from build123d import *

# Parameters (mm, degrees)
SKETCH1_R           = 0.5
SKETCH1_R_2         = 1.695720035
SKETCH1_W           = 3.739481929
SKETCH1_H           = 1.068423409
SKETCH1_W_2         = 3.73948193
BOSS_EXTRUDE1_DEPTH = 4


with BuildPart() as part:
    # Sketch1 → Boss-Extrude1 (new body)
    with BuildSketch(Plane(origin=(0, 0, 0), x_dir=(1, 0, 0), z_dir=(0, 1, 0))):
        with BuildLine():
            Line((43.455785529, -19.365174275), (43.455785529, 24.440185465))
            Line((43.455785529, 24.440185465), (39.576612996, 24.440185465))
            Line((39.576612996, 24.440185465), (39.576612996, 12.960768953))
            Line((39.576612996, 12.960768953), (19.950470546, 12.960768953))
            Line((19.950470546, 12.960768953), (19.950470546, 24.039526687))
            Line((19.950470546, 24.039526687), (-11.673190701, 24.438144265))
            ThreePointArc((-11.673190701, 24.438144265), (-5.411187986, 17.934763274), (-11.83512585, 11.591289096))
            Line((-11.83512585, 11.591289096), (-30.532535496, 11.591289096))
            ThreePointArc((-30.532535496, 11.591289096), (-36.95698368, 18.01573728), (-30.532535496, 24.440185465))
            Line((-30.532535496, 24.440185465), (-37.72291673, 24.440185465))
            Line((-37.72291673, 24.440185465), (-37.72291673, -19.365174275))
            Line((-37.72291673, -19.365174275), (-30.532535496, -19.365174275))
            ThreePointArc((-30.532535496, -19.365174275), (-37.109148108, -12.788561662), (-30.532535496, -6.21194905))
            Line((-30.532535496, -6.21194905), (-11.83512585, -6.21194905))
            ThreePointArc((-11.83512585, -6.21194905), (-5.258513237, -12.788561662), (-11.83512585, -19.365174275))
            Line((-11.83512585, -19.365174275), (20.193370142, -19.365174275))
            Line((20.193370142, -19.365174275), (20.193370142, -7.879622636))
            Line((20.193370142, -7.879622636), (39.959203195, -7.879622636))
            Line((39.959203195, -7.879622636), (39.959203195, -19.365174275))
            Line((39.959203195, -19.365174275), (43.455785529, -19.365174275))
        make_face()
        with Locations((-21.183830673, -3.926210212)):
            Circle(SKETCH1_R, mode=Mode.SUBTRACT)
        with Locations((-21.183830673, 2.537505595)):
            Circle(SKETCH1_R_2, mode=Mode.SUBTRACT)
        with Locations((17.397892673, 2.537505595)):
            Circle(SKETCH1_R, mode=Mode.SUBTRACT)
        with Locations((29.229431853, -4.460421917)):
            Rectangle(SKETCH1_W, SKETCH1_H, mode=Mode.SUBTRACT)
        with Locations((27.359690888, 2.537505595)):
            Circle(SKETCH1_R, mode=Mode.SUBTRACT)
        with Locations((-21.183830673, 8.146728488)):
            Circle(SKETCH1_R, mode=Mode.SUBTRACT)
        with Locations((29.299175369, 8.680940192)):
            Rectangle(SKETCH1_W_2, SKETCH1_H, mode=Mode.SUBTRACT)
    extrude(amount=BOSS_EXTRUDE1_DEPTH)


solid = part.part
Check sheet for the modelled part. Datum: model origin and axes. Units: mm. A direction names the side the tool comes from. Give positions to 0.01 mm unless a question says otherwise; leave off trailing zeros. Loops run counter-clockwise (first coordinate to the right, second up) from the corner with the lowest first, then second, coordinate; pieces in that order, holes last. Notation, with made-up numbers: M 41,-21.5 L 93,-21.5 A19 cw 93,-16.5 Z; hole C -18,-4.5 d4. An arc over 180 degrees is marked long. Return JSON: item names as keys, results as strings. Group by question number.
1. Cross-section at A-A on x = 29.5. Record the boundary of the cut face in (y, z), plus the area to 3 significant figures.
2. Cross-section at C-C on y = 1.9. State how many separate pieces and enclosed holes the cut face has, plus the area to 3 significant figures.
3. Go/stop test with flat-tipped pins: pin 1 (4 mm diameter, centred on x = -22.5, z = -14.5, fed in from +Y); pin 2 (1.9 mm diameter, centred on x = 30, y = 2.5, fed in from -Z); pin 3 (1.9 mm diameter, centred on x = 29, y = 2.5, fed in from +Z); pin 4 (1.2 mm diameter, centred on x = -20.5, y = 1.5, fed in from -Z). Record where each tip stops, or that it passes through.
4. Mould release check, pull along X, two halves, no side actions. Record for faces 1 (the flat face through (-37.723, 2, -3)), 2 (the flat face through (-21, 2, 6.212)), 3 (the flat face through (2, 4, -3)): released by +X, released by -X, zero draft, split by the parting line, or undercut.
5. Cross-section at D-D on x = -13. Record the boundary of the cut face in (y, z), plus the area to 3 significant figures.
6. Cross-section at B-B on z = 10. Record the boundary of the cut face in (x, y), plus the area to 3 significant figures.
7. Tool access check on faces 4 (the flat face through (19.95, 2, -18)), 5 (the cylindrical face through (-36.955, 1.972, -17.874)), 6 (the flat face through (30, 2, 7.88)), 7 (the flat face through (-34, 2, -24.44)), 8 (the flat face through (2, 0, -3)). Record the directions out of +Z, -Z, +X, -X, +Y, -Y that give a thin tool (end or side, any length) a straight path to the whole face; none if there is none.
8. Thickness scan on L1, parallel to X at y = 1.8, z = 12.5; L2, parallel to Z at x = 27.5, y = 3.25; L3, parallel to X at y = 2.2, z = -22. Record the ranges inside material, lowest first.
Return value:
{
 "1": {"outline": "M 0,-12.96 L 4,-12.96 L 4,-9.22 L 0,-9.22 Z; M 0,-8.15 L 4,-8.15 L 4,3.93 L 0,3.93 Z; M 0,4.99 L 4,4.99 L 4,7.88 L 0,7.88 Z", "area": "74.8 mm^2"},
 "2": {"separate pieces": "1", "enclosed holes": "7", "area": "2,330 mm^2"},
 "3": {"pin 1": "through", "pin 2": "z = -12.96", "pin 3": "z = 7.88", "pin 4": "z = -11.59"},
 "4": {"face 1": "released by -X", "face 2": "undercut", "face 3": "zero draft"},
 "5": {"outline": "M 0,-11.59 L 4,-11.59 L 4,6.21 L 0,6.21 Z", "area": "71.2 mm^2"},
 "6": {"outline": "M -37.72,0 L -36.49,0 L -36.49,4 L -37.72,4 Z; M -5.88,0 L 20.19,0 L 20.19,4 L -5.88,4 Z; M 39.96,0 L 43.46,0 L 43.46,4 L 39.96,4 Z", "area": "123 mm^2"},
 "7": {"face 4": "-Z, +Y, -Y", "face 5": "+Y, -Y", "face 6": "+Z, +Y, -Y", "face 7": "-Z, +X, -X, +Y, -Y", "face 8": "+Z, -Z, +X, -X, -Y"},
 "8": {"L1": "-37.72 to -37.1, -5.26 to 20.19, 39.96 to 43.46", "L2": "-12.96 to -9.22, -8.15 to -3.02, -2.06 to 3.93, 4.99 to 7.88", "L3": "-37.72 to -35.57, -6.8 to 19.95, 39.58 to 43.46"}
}
